The listing builds one solid part. Answer for the finished solid, in the listing's coordinates (mm). Give positions to 0.01 mm unless a question says otherwise; leave off trailing zeros. Order: outer loops, then holes, each group sorted by start corner. A loop starts at its lowest first (then second) coordinate and runs counter-clockwise, first axis right, second up.
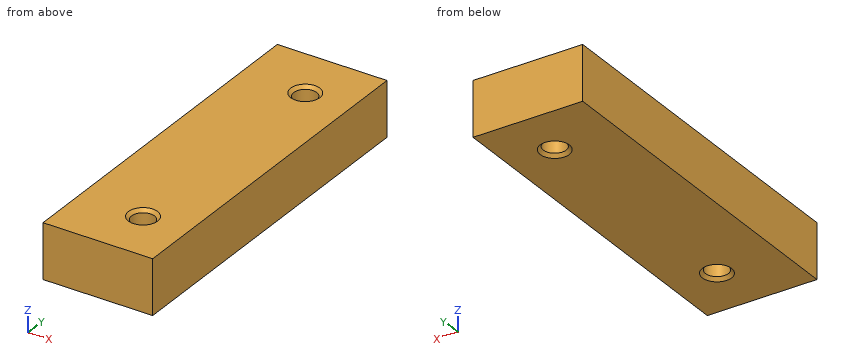
```python
from build123d import *

# Parameters (mm, degrees)
SKETCH_1_W                 = 12
SKETCH_1_H                 = 6
EXTRUDE_1_DEPTH            = 39
HOLE_WIZARD_M31_AT_2_COUNT = 2
HOLE_WIZARD_M31_AT_2_PITCH = 27


with BuildPart() as part:
    # Эскиз1 → Бобышка-Вытянуть1 (new body)
    with BuildSketch(Plane(origin=(0, 0, 0), x_dir=(1, 0, 0), z_dir=(0, 1, 0))):
        with Locations((6, 3)):
            Rectangle(SKETCH_1_W, SKETCH_1_H)
    extrude(amount=EXTRUDE_1_DEPTH)

    # Эскиз2 → Отверстие обработанное метчиком M31 (revolve, cut)
    with BuildSketch(Plane(origin=(7, 6, 0), x_dir=(0, -1, 0), z_dir=(1, 0, 0))):
        Polygon((0, 0), (0, 6), (1.6, 6), (1.25, 5.65), (1.25, 0.35), (1.6, 0), align=None)
    hole_wizard_m31 = revolve(axis=Axis((7, 6, 6.35), (0, 0, -1)), mode=Mode.SUBTRACT)

    # Отверстие обработанное метчиком M31 at 2: Отверстие обработанное метчиком M31 ×2
    with Locations(*[(0, i * HOLE_WIZARD_M31_AT_2_PITCH, 0) for i in range(1, HOLE_WIZARD_M31_AT_2_COUNT)]):
        add(hole_wizard_m31, mode=Mode.SUBTRACT)


solid = part.part
```
1) Find section B-B (y = 33). Write down the section's boundary in (x, z), then the cut area to 3 significant figures.
Geometry says:
outline: (0, -6) - (5.4, -6) - (5.75, -5.65) - (5.75, -0.35) - (5.4, 0) - (0, 0) - close; (8.25, -5.65) - (8.6, -6) - (12, -6) - (12, 0) - (8.6, 0) - (8.25, -0.35) - close
area: 56.8 mm2
2) Straight lines are drawn through the part: probe 1 along Y at (x, z) = (7, -3.35); probe 2 along X at (y, z) = (33, -1.95); probe 3 along Y at (x, z) = (6.5, -4.7). For each, find the intervals that lie inside material, in ascending order.
Geometry says:
probe 1: y = 0 to 4.75, 7.25 to 31.75, 34.25 to 39
probe 2: x = 0 to 5.75, 8.25 to 12
probe 3: y = 0 to 4.85, 7.15 to 31.85, 34.15 to 39
3) Given P1, Ø3, axis at x = 7, y = 6, coming from the +Z side, flat-ended and moving along its own axis, determine where the tip first touches the part or whether it passes through.
Geometry says:
P1: stops at z = -0.1
4) Find section A-A (x = 7). Write down the section's boundary in (y, z).
Geometry says:
outline: (0, -6) - (4.4, -6) - (4.75, -5.65) - (4.75, -0.35) - (4.4, 0) - (0, 0) - close; (7.25, -5.65) - (7.6, -6) - (31.4, -6) - (31.75, -5.65) - (31.75, -0.35) - (31.4, 0) - (7.6, 0) - (7.25, -0.35) - close; (34.25, -5.65) - (34.6, -6) - (39, -6) - (39, 0) - (34.6, 0) - (34.25, -0.35) - close
5) Find section C-C (z = -3.95). Write down the section's boundary in (x, y), then the cut area to 3 significant figures.
Geometry says:
outline: (0, 0) - (12, 0) - (12, 39) - (0, 39) - close; hole circle Ø2.5 at (7, 6); hole circle Ø2.5 at (7, 33)
area: 458 mm2
